```python
from build123d import *

# Parameters (mm, degrees)
F0_R     = 5
F1_DEPTH = 10


with BuildPart() as f1:
    # F0 (on Top) → F1 (new body)
    with BuildSketch(Plane.XY):
        Circle(F0_R)
        Polygon((0.578808, 3.654447), (0, 0), (-0.578808, 3.654447), (0, 3.9), align=None, mode=Mode.SUBTRACT)
    extrude(amount=F1_DEPTH)


solid = f1.part
```
Work out the finished part from the listing and answer in its coordinate system (mm). A direction names the side the tool comes from. Round coordinates to 2 decimals unless told otherwise and drop trailing zeros. Loops run counter-clockwise (first coordinate to the right, second up) from the corner with the lowest first, then second, coordinate; pieces in that order, holes last. Notation, with made-up numbers: M 17.25,-13.75 L 35.25,-13.75 A9 ccw 35.25,3.25 Z; hole C 59.25,78 d9. An arc over 180 degrees is marked long. Use CSV: the item, a comma, the result in double quotes.
Q1. Section B-B, the plane z = 6.5 is taken. Determine the outline of the cut face in (x, y).
Determined:
outline,"C 0,0 d10; hole M -0.58,3.65 L 0,0 L 0.58,3.65 L 0,3.9 Z"
Q2. Each of these flat-tipped pins is pushed along its axis until it touches: pin 1 (2 mm diameter, centred on y = -2.5, z = 5, fed in from -X); pin 2 (1 mm diameter, centred on x = 4, z = 2.5, fed in from -Y); pin 3 (6 mm diameter, centred on x = -3.5, z = 5.5, fed in from -Y). Where does it stop, or does it pass through?
Determined:
pin 1,"x = -4.77"
pin 2,"y = -3.57"
pin 3,"y = -4.97"
Q3. Section A-A, the plane y = 2.5 is taken. Determine the outline of the cut face in (x, z), then the cut area to 3 significant figures.
Determined:
outline,"M -4.33,0 L -0.4,0 L -0.4,10 L -4.33,10 Z; M 0.4,0 L 4.33,0 L 4.33,10 L 0.4,10 Z"
area,"78.7 mm2"
Q4. Section C-C, the plane y = 0.5 is taken. Determine the outline of the cut face in (x, z).
Determined:
outline,"M -4.97,0 L -0.08,0 L -0.08,10 L -4.97,10 Z; M 0.08,0 L 4.97,0 L 4.97,10 L 0.08,10 Z"
Q5. The mould has two halves that part along X. Classify faces 1 (the flat face through (0.3, 1.9, 4.9)), 2 (the cylindrical face through (-1.08, -4.88, 4.93)), 3 (the flat face through (0, -1, 10)): pulls with the +X half, pulls with the -X half, needs draft (parallel to the pull), parting line crosses it, or undercut.
Determined:
face 1,"undercut"
face 2,"parting line crosses it"
face 3,"needs draft"
Q6. Consider L1, parallel to X at y = 2.25, z = 7.25; L2, parallel to X at y = 3.75, z = 5.75; L3, parallel to X at y = 4.5, z = 6. Determine where each line is inside the solid, lowest interval first.
Determined:
L1,"-4.47 to -0.36, 0.36 to 4.47"
L2,"-3.31 to -0.35, 0.35 to 3.31"
L3,"-2.18 to 2.18"
Q7. A tool of negligible diameter and unlimited length cuts with its end or side. For faces 4 (the flat face through (-0.285, 1.802, 4.93)), 5 (the flat face through (0, -1, 0)), from which of +Z, -Z, +X, -X, +Y, -Y can it reach the whole face along a straight path? Write none if from no direction.
Determined:
face 4,"+Z, -Z"
face 5,"-Z, +X, -X, +Y, -Y"
Q8. Section D-D, the plane x = 2 is taken. Determine the outline of the cut face in (y, z), then the cut area to 3 significant figures.
Determined:
outline,"M -4.58,0 L 4.58,0 L 4.58,10 L -4.58,10 Z"
area,"91.7 mm2"
